Part print with two shaded views. Sizes in mm from the minimum x, y, z corner. A direction names the side the tool comes from. Give positions to 0.01 mm unless a question says otherwise; leave off trailing zeros. Write each loop counter-clockwise with the first axis right and the second up, starting at its lowest first coordinate (ties: lowest second). Pieces come first, ordered by that corner, then holes.
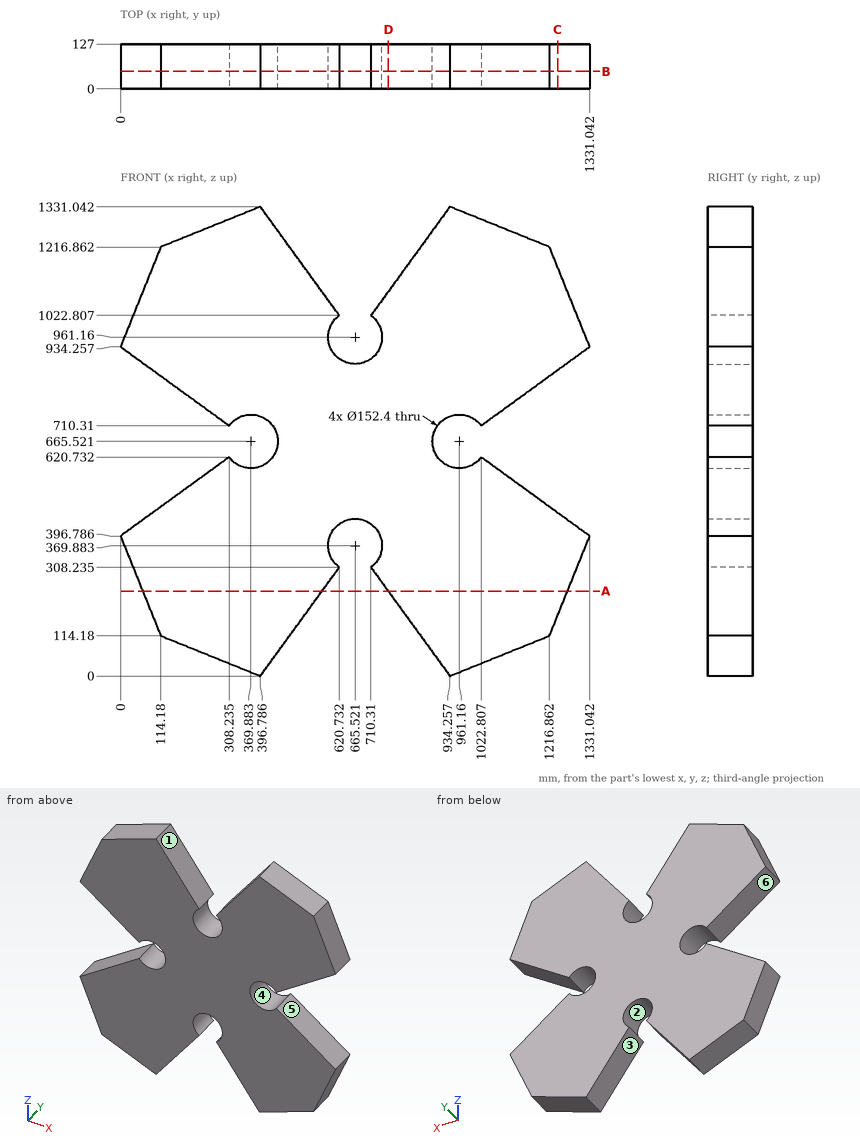
1) Pin check, flat tips, straight feed: pin 1 Ø12 at (y, z) = (60, 603.5) entering from +X (1 decimal); pin 2 Ø5 at (x, y) = (224.5, 100.5) entering from +Z (1 decimal); pin 3 Ø2 at (y, z) = (112.5, 457) entering from +X. Stop position of each tip, or through.
Answers follow:
pin 1: stops at x = 1054.8
pin 2: stops at z = 1262.4
pin 3: stops at x = 1249.54
2) Two-plate mould, pull along X, no slides. Class the marked faces 4, 5 and 6: +X half, -X half, draft (parallel to the pull), parting line (faces both ways), or undercut.
Answers follow:
face 4: undercut
face 5: +X half
face 6: -X half
3) Saw through at C-C, the plane x = 1240. Write the cut outline in (y, z) (1 decimal), then the cut area to 3 significant figures.
Answers follow:
outline: (0, 171.4) - (127, 171.4) - (127, 462.9) - (0, 462.9) - close; (0, 868.1) - (127, 868.1) - (127, 1159.6) - (0, 1159.6) - close
area: 74,000 mm2
4) 3-axis set-ups, long thin cutter, end or side, ignore diameter. For the marked faces 1, 2 and 3: which of +Z, -Z, +X, -X, +Y, -Y reach the whole face in a straight line?
Answers follow:
face 1: +Z, +Y, -Y
face 2: +Y, -Y
face 3: -Z, +Y, -Y
5) Saw through at B-B, the plane y = 49.5. Write the cut outline in (x, z) (1 decimal).
Answers follow:
outline: (0, 396.8) - (114.2, 114.2) - (396.8, 0) - (620.7, 308.2) arc R76.2 cw (long way) to (710.3, 308.2) - (934.3, 0) - (1216.9, 114.2) - (1331, 396.8) - (1022.8, 620.7) arc R76.2 cw (long way) to (1022.8, 710.3) - (1331, 934.3) - (1216.9, 1216.9) - (934.3, 1331) - (710.3, 1022.8) arc R76.2 cw (long way) to (620.7, 1022.8) - (396.8, 1331) - (114.2, 1216.9) - (0, 934.3) - (308.2, 710.3) arc R76.2 cw (long way) to (308.2, 620.7) - close
6) Wall check: L1, parallel to X at y = 54, z = 601 (1 decimal); L2, parallel to X at y = 24.5, z = 660.5 (1 decimal); L3, parallel to X at y = 95.5, z = 320 (1 decimal). Give the ranges that are in metal, low to high.
Answers follow:
L1: x = 281.1 to 329.3, 410.4 to 920.6, 1001.7 to 1050
L2: x = 445.9 to 885.1
L3: x = 31 to 607.9, 723.1 to 1300
7) Saw through at D-D, the plane x = 760. Write the cut outline in (y, z), then the cut area to 3 significant figures.
Answers follow:
outline: (0, 239.84) - (127, 239.84) - (127, 1091.2) - (0, 1091.2) - close
area: 108,000 mm2
8) Saw through at A-A, the plane z = 240.5. Write the cut outline in (x, y), then the cut area to 3 significant figures.
Answers follow:
outline: (63.14, 0) - (571.52, 0) - (571.52, 127) - (63.14, 127) - close; (759.52, 0) - (1267.9, 0) - (1267.9, 127) - (759.52, 127) - close
area: 129,000 mm2
